Geometry: final body of the model. Coordinates: model frame, mm. A direction names the side the tool comes from. Coordinates: 2 decimals unless noted, no trailing zeros. Write each loop counter-clockwise with the first axis right and the second up, starting at its lowest first coordinate (ties: lowest second). Pieces come first, ordered by that corner, then holes.
Autodesk Fusion 360 part; units mm, degrees
sketch "Sketch1" plane through (0, 0, 0) normal (1, 0, 0) x (0, 1, 0)
  line L0 (0, 0) -> (25.696, 0)
  line L1 (25.696, 0) -> (25.696, 25)
  line L2 (25.696, 25) -> (0, 25)
  line L3 (0, 25) -> (0, 0)
  dimension "d1" = 25.696
  dimension "d2" = 25
extrude "Extrude1" add sketch "Sketch1" along normal blind 3.046
sketch "Sketch4" plane through (3.046, 0, 0) normal (1, 0, 0) x (0, 1, 0)
  line L0 (0, 25) -> (0, 0)
  line L1 (0, 0) -> (25.696, 0)
  line L2 (25.696, 0) -> (25.696, 25)
  line L3 (25.696, 25) -> (0, 25)
  line L4 (0, 0) -> (0.696, 0)
  line L5 (0.696, 0) -> (0.696, 25)
  line L6 (0.696, 25) -> (0, 25)
  line L7 (0, 25) -> (0, 0)
  line L8 (12.848, 25) -> (12.848, 0) construction
  line L9 (25.696, 25) -> (25.696, 0)
  line L10 (25, 0) -> (25, 25)
  dimension "d15" = 0.696
  dimension "d16" = 25
extrude "Extrude3" add sketch "Sketch4" along normal blind 4.8 and the other way blind 10.6 contours L0 L1 L3 L4 L5 L6 L7 | L1 L2 L3 L9 L10
sketch "Sketch5" plane through (3.046, 0, 0) normal (1, 0, 0) x (0, 1, 0)
  line L0 (25, 0) -> (25, 25)
  line L1 (25, 25) -> (0.696, 25)
  line L2 (0.696, 25) -> (0.696, 0)
  line L3 (0.696, 0) -> (25, 0)
  line L4 (4.63, 25) -> (4.63, 0)
  line L5 (5.294, 25) -> (5.294, 0)
  line L6 (9.63, 25) -> (9.63, 0)
  line L7 (10.294, 25) -> (10.294, 0)
  line L8 (12.848, 25) -> (12.848, 0) construction
  line L9 (21.066, 25) -> (21.066, 0)
  line L10 (20.402, 25) -> (20.402, 0)
  line L11 (16.066, 25) -> (16.066, 0)
  line L12 (15.402, 25) -> (15.402, 0)
  dimension "d21" = -3.934
  dimension "d22" = -4.598
  dimension "d23" = -8.934
  dimension "d24" = -9.598
extrude "Extrude4" add sketch "Sketch5" along normal blind 4.8 contours L1 L3 L9 L10 | L1 L3 L11 L12 | L1 L3 L6 L7 | L1 L3 L4 L5
sketch "Sketch6" plane through (0, 0, 0) normal (0, 0, 1) x (1, 0, 0)
  circle A0 centre (2.4572, 2.6766) radius 1
  line L0 (0, 0) -> (0, 25.696)
  line L1 (0, 12.848) -> (3.046, 12.848) construction
  circle A1 centre (2.4572, 23.0194) radius 1
  dimension "d27" = 2
  dimension "d28" = 25.696
  dimension "d29" = 3.046
extrude "Extrude5" cut sketch "Sketch6" along normal blind 25
sketch "Sketch7" plane through (0, 0, 0) normal (1, 0, 0) x (0, 1, 0)
sketch "Sketch8" plane through (3.046, 0, 0) normal (1, 0, 0) x (0, 1, 0)
  line L0 (15.402, 0) -> (15.402, 25)
  line L1 (15.402, 25) -> (10.294, 25)
  line L2 (10.294, 25) -> (10.294, 0)
  line L3 (10.294, 0) -> (15.402, 0)
  line L4 (12.848, 0) -> (12.848, 17) construction
  circle A0 centre (12.848, 17) radius 1.75
  dimension "d32" = 3.5
extrude "Extrude6" cut sketch "Sketch8" against normal blind 3.046 contours A0
sketch "Sketch9" plane through (0, 0, 0) normal (0, 0, 1) x (1, 0, 0)
sketch "Sketch10" plane through (0, 0, 0) normal (1, 0, 0) x (0, 1, 0)
extrude "Extrude7" cut 1 faces at (3.046, 8.1847, 8.3333) along direction (-1, 0, 0) blind 1.5
sketch "Sketch11" plane through (0, 0, 0) normal (1, 0, 0) x (0, 1, 0)
extrude "Extrude8" cut 1 faces at (3.046, 17.5113, 8.3333) along direction (-1, 0, 0) blind 1.5
fillet "Fillet1" radius 0.4 10 edges at (3.046, 0.696, 12.5) (3.046, 4.63, 12.5) (1.546, 9.63, 12.5) (3.046, 15.402, 12.5) (1.546, 20.402, 12.5) (3.046, 25, 12.5) (1.546, 5.294, 12.5) (3.046, 10.294, 12.5) (1.546, 16.066, 12.5) (3.046, 21.066, 12.5)
fillet "Fillet2" radius 0.4 2 edges at (0, 25, 12.5) (0, 0.696, 12.5)
sketch "Sketch12" plane through (0, 0, 0) normal (1, 0, 0) x (0, 1, 0)
  line L0 (25.696, 25) -> (25.696, 0)
  circle A0 centre (12.848, 17) radius 1.75
  dimension "d45" = 25
  dimension "d46" = 25.696
  dimension "d47" = 3.5
sketch "Sketch13" plane through (0, 0, 0) normal (0, 1, 0) x (1, 0, 0)
  line L0 (7.846, -25) -> (7.846, 0)
  line L1 (-7.554, 0) -> (7.846, 0)
  dimension "d48" = 25
  dimension "d49" = 15.4
sketch "Sketch14" plane through (0, 0, 0) normal (0, 0, 1) x (1, 0, 0)
  arc A0 (3.046, 3.4849) -> (3.046, 1.8683) centre (2.4572, 2.6766) ccw
  line L0 (3.446, 4.63) -> (7.846, 4.63)
  line L1 (7.846, 5.294) -> (1.946, 5.294)
  line L2 (1.546, 5.694) -> (1.546, 9.23)
  line L3 (3.046, 15.002) -> (3.046, 10.694)
  line L4 (3.446, 10.294) -> (7.846, 10.294)
  line L5 (3.446, 0.696) -> (7.846, 0.696)
  point P0 (-7.554, 0)
  point P1 (-7.554, 25.696)
  dimension "d50" = 25.696
  dimension "d51" = 1
  dimension "d53" = 5.9
  dimension "d54" = 3.536
  dimension "d55" = 4.308
  dimension "d56" = 4.4
  dimension "d57" = 4.4
sketch "Sketch15" plane through (0, 0, 0) normal (1, 0, 0) x (0, 1, 0)
  line L0 (9.63, 25) -> (9.63, 0)
  dimension "d58" = 25
equation "d6 = -0.696 mm - 3.934 mm"
equation "d7 = -0.696 mm - 3.934 mm - 0.664 mm"
equation "d8 = -0.696 mm - 3.934 mm - 0.664 mm - 4.336 mm"
equation "d9 = -0.696 mm - 3.934 mm - 0.664 mm - 4.336 mm - 0.664 mm"
equation "d19 = 3.046 mm + 7.554 mm"
equation "d22 = -3.934 mm - 0.664 mm"
equation "d23 = -3.934 mm - 0.664 mm - 4.336 mm"
equation "d24 = -3.934 mm - 0.664 mm - 4.336 mm - 0.664 mm"
Item 1: Section A-A, the plane x = 4.25. Output: boundary loops of the cut face in (y, z).
Derived:
outline: (0, 0) - (0.7, 0) - (0.7, 25) - (0, 25) - close; (4.63, 0) - (5.29, 0) - (5.29, 25) - (4.63, 25) - close; (9.63, 0) - (10.29, 0) - (10.29, 25) - (9.63, 25) - close; (15.4, 0) - (16.07, 0) - (16.07, 25) - (15.4, 25) - close; (20.4, 0) - (21.07, 0) - (21.07, 25) - (20.4, 25) - close; (25, 0) - (25.7, 0) - (25.7, 25) - (25, 25) - close
Item 2: Section B-B, the plane x = -2.5. Output: boundary loops of the cut face in (y, z), plus the area to 3 significant figures.
Derived:
outline: (0, 0) - (0.7, 0) - (0.7, 25) - (0, 25) - close; (25, 0) - (25.7, 0) - (25.7, 25) - (25, 25) - close
area: 34.8 mm2
Item 3: Pull-direction query (Z, two-part tool) for faces 4 (the flat face through (0, 25.696, 12)), 5 (the cylindrical face through (1.544, 12.62, 18.735)), 6 (the flat face through (2, 13, 0)), 7 (the flat face through (2, 13, 25)); classes: released by +Z, released by -Z, zero draft, split by the parting line, or undercut.
Derived:
face 4: zero draft
face 5: undercut
face 6: released by -Z
face 7: released by +Z
Item 4: Material intervals for probe 1 along Y at (x, z) = (3.5, 21.75); probe 2 along Y at (x, z) = (-1.25, 16.75); probe 3 along X at (y, z) = (19.75, 22.25), sorted ascending.
Derived:
probe 1: y = 0 to 0.7, 4.63 to 5.29, 9.63 to 10.29, 15.4 to 16.07, 20.4 to 21.07, 25 to 25.7
probe 2: y = 0 to 0.7, 25 to 25.7
probe 3: x = 0 to 1.55
Item 5: Section C-C, the plane y = 15.75. Output: boundary loops of the cut face in (x, z), plus the area to 3 significant figures.
Derived:
outline: (0, 0) - (7.85, 0) - (7.85, 25) - (0, 25) - close
area: 196 mm2
Item 6: Pin query (flat end, axial travel): pin 1 (8 mm diameter, centred on y = 11.5, z = 6.5, fed in from -X); pin 2 (1.6 mm diameter, centred on x = 2.46, y = 2.68, fed in from +Z). Return the tip coordinate at first contact, or that it passes through.
Derived:
pin 1: stops at x = 0
pin 2: passes through
Item 7: Set-up query: faces 1 (the flat face through (0, 0, 13)), 2 (the flat face through (6, 4.63, 13)), 3 (the flat face through (0, 13, 13)). Return all of +Z, -Z, +X, -X, +Y, -Y with unobstructed straight access to the full face (end or side cutting, diameter ignored); none if empty.
Derived:
face 1: +Z, -Z, +X, -X, -Y
face 2: +Z, -Z, +X
face 3: +Z, -Z, -X
